from build123d import *

# Parameters (mm, degrees)
F3_DEPTH = 140.001
F4_R     = 8
F5_DEPTH = 140.001
F6_R     = 4
F7_DEPTH = 90.001


with BuildPart() as f1:
    # F0 (on Front) → F1 (revolve)
    with BuildSketch(Plane.XZ):
        Polygon((28.6, 140), (28.6, 0), (60, 0), (60, 100), (90, 100), (90, 140), align=None)
    revolve(axis=Axis((0, 0, 42.943615), (0, 0, 1)))

    # F2 (on face) → F3 (cut, through all)
    with BuildSketch(Plane.XY.offset(140)):
        with BuildLine():
            Line((8, 33.4), (-8, 33.4))
            Line((-8, 33.4), (-8, 27.458332))
            ThreePointArc((-8, 27.458332), (0, 28.6), (8, 27.458332))
            Line((8, 27.458332), (8, 33.4))
        make_face()
    extrude(amount=-F3_DEPTH, mode=Mode.SUBTRACT)

    # F4 (on face) → F5 (cut, through all)
    with BuildSketch(Plane.XY.offset(140)):
        with Locations((-55.154329, 55.154329)):
            Circle(F4_R)
        with Locations((0, 78)):
            Circle(F4_R)
        with Locations((55.154329, 55.154329)):
            Circle(F4_R)
        with Locations((78, 0)):
            Circle(F4_R)
        with Locations((55.154329, -55.154329)):
            Circle(F4_R)
        with Locations((0, -78)):
            Circle(F4_R)
        with Locations((-55.154329, -55.154329)):
            Circle(F4_R)
        with Locations((-78, 0)):
            Circle(F4_R)
    extrude(amount=-F5_DEPTH, mode=Mode.SUBTRACT)

    # F6 (on Front) → F7 (cut, through all)
    with BuildSketch(Plane.XZ):
        with Locations((0, 50)):
            Circle(F6_R)
    extrude(amount=-F7_DEPTH, mode=Mode.SUBTRACT)


solid = f1.part
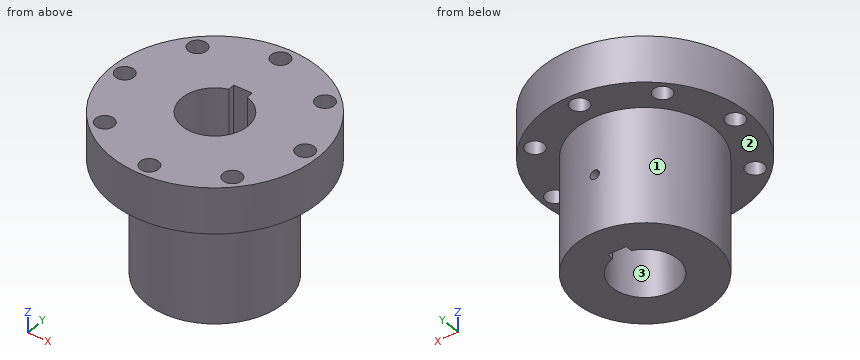
CAD build for the part. Positions are in the model's coordinates, mm. Face numbers are marked on the shaded views. Give positions to 0.01 mm unless a question says otherwise; leave off trailing zeros. Order: outer loops, then holes, each group sorted by start corner. A loop starts at its lowest first (then second) coordinate and runs counter-clockwise, first axis right, second up. Notation, with made-up numbers: (-10, 16.5) -> (22, 16.5) arc R12 cw to (22, 22.5) -> close; hole circle Ø4 at (57, 87). An arc over 180 degrees is marked (long way). Return JSON: item names as keys, results as strings.
Q1. Saw through at A-A (x = 0). Write the cut outline in (y, z), then the cut area to 3 significant figures.
Working result:
{"outline": "(-90, 100) -> (-86, 100) -> (-86, 140) -> (-90, 140) -> close; (-70, 100) -> (-60, 100) -> (-60, 0) -> (-28.6, 0) -> (-28.6, 140) -> (-70, 140) -> close; (33.4, 0) -> (60, 0) -> (60, 46) -> (33.4, 46) -> close; (33.4, 54) -> (60, 54) -> (60, 100) -> (70, 100) -> (70, 140) -> (33.4, 140) -> close; (86, 100) -> (90, 100) -> (90, 140) -> (86, 140) -> close", "area": "9,030 mm²"}
Q2. Flat gauge pins, fed straight in: pin 1 (17.5 mm diameter, centred on x = 1, z = 86, fed in from -Y); pin 2 (2 mm diameter, centred on x = -45, z = 20.5, fed in from +Y); pin 3 (2 mm diameter, centred on x = 56.5, z = 17, fed in from -Y); pin 4 (9.5 mm diameter, centred on x = 55.15, y = 55.15, fed in from -Z). Where does each tip first touch, or does it go through?
Working result:
{"pin 1": "y = -60", "pin 2": "y = 40.79", "pin 3": "y = -22.8", "pin 4": "through"}
Q3. Saw through at C-C (z = 59.5). Write the cut outline in (x, y), then the cut area to 3 significant figures.
Working result:
{"outline": "circle Ø120 at (0, 0); hole (-8, 27.46) arc R28.6 ccw (long way) to (8, 27.46) -> (8, 33.4) -> (-8, 33.4) -> close", "area": "8,660 mm²"}
Q4. Saw through at D-D (x = 73). Write the cut outline in (y, z) (3 decimals), then the cut area to 3 significant figures.
Working result:
{"outline": "(-52.64, 100) -> (-6.245, 100) -> (-6.245, 140) -> (-52.64, 140) -> close; (6.245, 100) -> (52.64, 100) -> (52.64, 140) -> (6.245, 140) -> close", "area": "3,710 mm²"}
Q5. Drill centre lines: line 1 (Y direction, x = 0, z = 106); line 2 (Z direction, x = 0, y = 50.5); line 3 (Y direction, x = 5, z = 103) (3 decimals). Where is each one in solid material? Low to high.
Working result:
{"line 1": "-90 to -86, -70 to -28.6, 33.4 to 70, 86 to 90", "line 2": "0 to 46, 54 to 140", "line 3": "-89.861 to -84.245, -71.755 to -28.16, 33.4 to 71.755, 84.245 to 89.861"}
Q6. Saw through at B-B (y = 0). Write the cut outline in (x, z).
Working result:
{"outline": "(-90, 100) -> (-86, 100) -> (-86, 140) -> (-90, 140) -> close; (-70, 100) -> (-60, 100) -> (-60, 0) -> (-28.6, 0) -> (-28.6, 140) -> (-70, 140) -> close; (28.6, 0) -> (60, 0) -> (60, 100) -> (70, 100) -> (70, 140) -> (28.6, 140) -> close; (86, 100) -> (90, 100) -> (90, 140) -> (86, 140) -> close"}
Q7. Mould opens along X. For the marked faces 1, 2 and 3 say: pulls with the +X half, pulls with the -X half, needs draft (parallel to the pull), parting line crosses it, or undercut.
Working result:
{"face 1": "parting line crosses it", "face 2": "needs draft", "face 3": "undercut"}
